Input: part model. Units: mm. Frame: model coordinates. A direction names the side the tool comes from. Give positions to 0.01 mm unless a question says otherwise; leave off trailing zeros. Loops run counter-clockwise (first coordinate to the right, second up) from the corner with the lowest first, then second, coordinate; pieces in that order, holes last. Notation, with made-up numbers: (11.25, 80) -> (48.25, 80) arc R25 cw to (48.25, 94) -> close; hole circle Ø9 at (41, 70.5). An arc over 180 degrees is marked (long way). Answer in a Markdown table with one row per item. Add a question column.
```python
from build123d import *

# Parameters (mm, degrees)
SKETCH_R             = 2.25
PAD_DEPTH            = 16
SKETCH002_W          = 116
SKETCH002_H          = 56
POCKET001_DEPTH      = 0.001
POCKET001_DEPTH_BACK = -16.001
SKETCH003_W          = 129
SKETCH003_H          = 62
POCKET002_DEPTH      = 6
SKETCH004_R          = 7.5
POCKET_DEPTH         = 8
SKETCH005_R          = 2.15
POCKET003_DEPTH      = 25


with BuildPart() as part:
    # Sketch → Pad (new body)
    with BuildSketch(Plane.XY):
        Polygon((87, 5), (302.6, 5), (302.6, 111.6), (166.6, 111.6), (166.6, 109.3), (162.9, 109.3), (162.9, 107.3), (168.6, 107.3), (168.6, 48), (87, 48), align=None)
        with Locations((292, 75.6)):
            Circle(SKETCH_R, mode=Mode.SUBTRACT)
    extrude(amount=PAD_DEPTH)

    # Sketch002 → Pocket001 (cut, two sides)
    with BuildSketch(Plane.XY) as pocket001_sk:
        with Locations((233.1, 38)):
            Rectangle(SKETCH002_W, SKETCH002_H)
    extrude(amount=-POCKET001_DEPTH, mode=Mode.SUBTRACT)
    extrude(pocket001_sk.sketch, amount=-POCKET001_DEPTH_BACK, mode=Mode.SUBTRACT)

    # Sketch003 (on DatumPlane) → Pocket002 (cut)
    with BuildSketch(Plane.XY.offset(24)):
        with Locations((233.1, 36)):
            Rectangle(SKETCH003_W, SKETCH003_H)
    extrude(amount=-POCKET002_DEPTH, mode=Mode.SUBTRACT)

    # Sketch004 → Pocket (cut)
    with BuildSketch(Plane.XY):
        with Locations((292, 75.6)):
            Circle(SKETCH004_R)
    extrude(amount=POCKET_DEPTH, mode=Mode.SUBTRACT)

    # Sketch005 → Pocket003 (cut)
    with BuildSketch(Plane.XZ):
        with Locations((296.2, 8)):
            Circle(SKETCH005_R)
    extrude(amount=-POCKET003_DEPTH, mode=Mode.SUBTRACT)


solid = part.part
```
1) Section B-B on x = 258. Output: boundary loops of the cut face in (y, z), and give its area (3 significant figures).
2) Section A-A on y = 15. Output: boundary loops of the cut face in (x, z).
3) Section C-C on y = 75.6. Output: boundary loops of the cut face in (x, z).
4) Reachability of faces 5 (the face through (232, 66, 8)), 6 (the face through (165, 109.3, 8)), 7 (the face through (286.048, 71.036, 3.944)) from +Z, -Z, +X, -X, +Y, -Y: full face, straight path, thin tool, end or side. Return the list, or none.
5) Section D-D on z = 3. Output: boundary loops of the cut face in (x, y), and give its area (3 significant figures).
6) Pin query (flat end, axial travel): pin 1 (1.1 mm diameter, centred on y = 110, z = 10.5, fed in from -X); pin 2 (1 mm diameter, centred on y = 108.5, z = 9, fed in from -X); pin 3 (4.5 mm diameter, centred on x = 288.5, y = 73, fed in from -Z). Return the tip coordinate at first contact, or that it passes through.
7) Pull-direction query (X, two-part tool) for faces 1 (the face through (87, 27, 8)), 2 (the face through (298.186, 14.86, 7.177)), 3 (the face through (302.6, 58, 8)), 4 (the face through (193, 71, 16)); classes: +X half, -X half, draft (parallel to the pull), parting line (faces both ways), or undercut.
8) Material intervals for line 1 along X through (y, z) = (19.5, 3.25); line 2 along Z through (x, y) = (296.2, 20.25); line 3 along Y through (x, z) = (292, 5), sorted ascending.
Working result:
| question | item | result |
|---|---|---|
| 1 | outline | (5, 0) -> (10, 0) -> (10, 16) -> (5, 16) -> close; (66, 0) -> (111.6, 0) -> (111.6, 16) -> (66, 16) -> close |
| 1 | area | 810 mm2 |
| 2 | outline | (87, 0) -> (175.1, 0) -> (175.1, 16) -> (87, 16) -> close; (291.1, 0) -> (302.6, 0) -> (302.6, 16) -> (291.1, 16) -> close; hole circle Ø4.3 at (296.2, 8) |
| 3 | outline | (168.6, 0) -> (284.5, 0) -> (284.5, 8) -> (289.75, 8) -> (289.75, 16) -> (168.6, 16) -> close; (294.25, 8) -> (299.5, 8) -> (299.5, 0) -> (302.6, 0) -> (302.6, 16) -> (294.25, 16) -> close |
| 4 | face 5 | +Z, -Z |
| 4 | face 6 | +Z, -Z, -X, +Y |
| 4 | face 7 | -Z |
| 5 | outline | (87, 5) -> (302.6, 5) -> (302.6, 111.6) -> (166.6, 111.6) -> (166.6, 109.3) -> (162.9, 109.3) -> (162.9, 107.3) -> (168.6, 107.3) -> (168.6, 48) -> (87, 48) -> close; hole (175.1, 10) -> (291.1, 10) -> (291.1, 66) -> (175.1, 66) -> close; hole circle Ø15 at (292, 75.6) |
| 5 | area | 11,100 mm2 |
| 6 | pin 1 | stops at x = 166.6 |
| 6 | pin 2 | stops at x = 162.9 |
| 6 | pin 3 | stops at z = 8 |
| 7 | face 1 | -X half |
| 7 | face 2 | undercut |
| 7 | face 3 | +X half |
| 7 | face 4 | draft |
| 8 | line 1 | x = 87 to 175.1, 291.1 to 302.6 |
| 8 | line 2 | z = 0 to 5.85, 10.15 to 16 |
| 8 | line 3 | y = 5 to 68.1, 83.1 to 111.6 |
